from build123d import *

# Parameters (mm, degrees)
BOSS_EXTRUDE1_DEPTH = 31
SKETCH4_W           = 25
SKETCH4_H           = 15
CUT_EXTRUDE2_DEPTH  = 25
CUT_EXTRUDE4_DEPTH  = 11.5
SKETCH7_W           = 31
SKETCH7_H           = 1.7
BOSS_EXTRUDE3_DEPTH = 7
BOSS_EXTRUDE4_DEPTH = 7
LPATTERN1_COUNT     = 8
LPATTERN1_PITCH     = 3.6
SKETCH11_W          = 12
SKETCH11_H          = 4.5
BOSS_EXTRUDE5_DEPTH = 3.5
FILLET5_R           = 3
SKETCH12_W          = 12
SKETCH12_H          = 4.5
BOSS_EXTRUDE6_DEPTH = 4.5
CUT_EXTRUDE5_DEPTH  = 12


with BuildPart() as part:
    # Sketch1 → Boss-Extrude1 (new body)
    with BuildSketch(Plane.XY):
        Polygon((0, 0), (0, -30), (12, -30), (12, -20), (5, 0), align=None)
    extrude(amount=-BOSS_EXTRUDE1_DEPTH)

    # Sketch4 → Cut-Extrude2 (cut)
    with BuildSketch(Plane.ZY):
        with Locations((-15, -24.143402944)):
            Rectangle(SKETCH4_W, SKETCH4_H)
    extrude(amount=-CUT_EXTRUDE2_DEPTH, mode=Mode.SUBTRACT)

    # Sketch6 → Cut-Extrude4 (cut, symmetric)
    with BuildSketch(Plane.XY.offset(-15.25)):
        Polygon((5, 0), (5, -14), (9.9, -14), align=None)
    extrude(amount=CUT_EXTRUDE4_DEPTH, both=True, mode=Mode.SUBTRACT)

    # Sketch7 → Boss-Extrude3 (add)
    with BuildSketch(Plane(origin=(0, -27, 0), x_dir=(1, 0, 0), z_dir=(0, 1, 0))):
        with Locations((-4.2231607, 26.8)):
            Rectangle(SKETCH7_W, SKETCH7_H)
    extrude(amount=BOSS_EXTRUDE3_DEPTH)

    # Sketch10 → Boss-Extrude4 (add)
    with BuildSketch(Plane(origin=(0, -27, 0), x_dir=(1, 0, 0), z_dir=(0, 1, 0))):
        with BuildLine():
            Line((10.226247744, 22.144145979), (9.378053282, 22.144145979))
            ThreePointArc((9.378053282, 22.144145979), (8.729742796, 23.468564149), (8.93378471, 24.928960283))
            ThreePointArc((8.93378471, 24.928960283), (8.707970922, 25.446557347), (8.452150513, 25.95))
            Line((8.452150513, 25.95), (11.152150513, 25.95))
            ThreePointArc((11.152150513, 25.95), (10.896330104, 25.446557347), (10.670516315, 24.928960283))
            ThreePointArc((10.670516315, 24.928960283), (10.874558229, 23.468564149), (10.226247744, 22.144145979))
        make_face()
    boss_extrude4 = extrude(amount=BOSS_EXTRUDE4_DEPTH)

    # LPattern1: Boss-Extrude4 ×8
    with Locations(*[(-i * LPATTERN1_PITCH, 0, 0) for i in range(1, LPATTERN1_COUNT)]):
        add(boss_extrude4)

    # Sketch11 → Boss-Extrude5 (add)
    with BuildSketch(Plane(origin=(0, 0, -31), x_dir=(-1, 0, 0), z_dir=(0, 0, -1))):
        with Locations((-6, -27.75)):
            Rectangle(SKETCH11_W, SKETCH11_H)
    extrude(amount=BOSS_EXTRUDE5_DEPTH)

    # Fillet5
    fillet5_edges = [part.edges().sort_by_distance(p)[0] for p in [
        (5.412595515, -16.643402944, -27.5),
        (5.412595515, -16.643402944, -2.5),
        (5, -14, -15.25),
    ]]
    fillet(fillet5_edges, radius=FILLET5_R)

    # Sketch12 → Boss-Extrude6 (add)
    with BuildSketch(Plane.XY):
        with Locations((6, -27.75)):
            Rectangle(SKETCH12_W, SKETCH12_H)
    extrude(amount=BOSS_EXTRUDE6_DEPTH)

    # Sketch13 → Cut-Extrude5 (cut)
    with BuildSketch(Plane.ZY):
        Polygon((-33.25, -27.047861031), (-26.75, -27.047861031), (-26.75, -32.047861031), (-31.25, -32.047861031), (-31.25, -28.847861031), (-33.25, -28.847861031), align=None)
        Polygon((1.676178687, -28.847861031), (3.676178687, -28.847861031), (3.676178687, -27.047861031), (-2.823821313, -27.047861031), (-2.823821313, -32.047861031), (1.676178687, -32.047861031), align=None)
    extrude(amount=-CUT_EXTRUDE5_DEPTH, mode=Mode.SUBTRACT)


solid = part.part
Source: CAD feature listing. Evaluate the final solid. Frame: model axes, mm. A direction names the side the tool comes from. Round coordinates to 2 decimals unless told otherwise and drop trailing zeros. Loops run counter-clockwise (first coordinate to the right, second up) from the corner with the lowest first, then second, coordinate; pieces in that order, holes last. Notation, with made-up numbers: (25, 85) - (78, 85) arc R20 ccw to (78, 92) - close; hole circle Ø5 at (21, 12.5). An arc over 180 degrees is marked (long way). Write item = value, one per line. Start each with the question number.
(1) Ray query, line 1 along Z through (x, y) = (1, -20.75); line 2 along Z through (x, y) = (8, -11.5); line 3 along Y through (x, z) = (2, -21). Return the intervals inside material, ascending. Write a range as from..to.
(2) Pin query (flat end, axial travel): pin 1 (0.9 mm diameter, centred on x = -5, y = -24, fed in from +Z); pin 2 (2 mm diameter, centred on x = -1.5, y = -16.5, fed in from -Z) (3 decimals); pin 3 (1.5 mm diameter, centred on x = 7.5, y = -6, fed in from +Z); pin 4 (12 mm diameter, centred on y = -22, z = -18, fed in from -X). Return the tip coordinate at first contact, or that it passes through.
(3) Section query B-B, the plane z = -17. Output: boundary loops of the cut face in (x, y).
(4) Section query A-A, the plane y = -28. Output: boundary loops of the cut face in (x, z), plus the area to 3 significant figures.
(5) Set-up query: faces 1 (the face through (5, -5, -15)), 2 (the face through (6, -27.048, 1)), 3 (the face through (-16.49, -23.55, -25.44)). Return all of +Z, -Z, +X, -X, +Y, -Y with unobstructed straight access to the full face (end or side cutting, diameter ignored); none if empty.
(6) Pull-direction query (Z, two-part tool) for faces 4 (the face through (-10.722, -23.549, -23.489)), 5 (the face through (-10, -24, -27.65)), 6 (the face through (-13.6, -23.5, -25.95)), 7 (the face through (0, -12, -15)); classes: +Z half, -Z half, draft (parallel to the pull), parting line (faces both ways), or undercut.
(7) Section query C-C, the plane y = -9.25. Output: boundary loops of the cut face in (x, z), plus the area to 3 significant figures.
(8) Section query D-D, the plane y = -18.5. Output: boundary loops of the cut face in (x, z) (3 decimals).
Conclusion:
q1.line_1 = -31..-25.95, -2.5..0
q1.line_2 = -31..-26.75, -3.75..0
q1.line_3 = -16.64..0
q2.pin_1 = -22.14
q2.pin_2 = through
q2.pin_3 = 0
q2.pin_4 = -16.5
q3.outline = (0, -16.64) - (10.83, -16.64) - (9.9, -14) - (8, -14) arc R3 cw to (5, -11) - (5, 0) - (0, 0) - close
q4.outline = (0, -34.5) - (12, -34.5) - (12, -33.25) - (0, -33.25) - close; (0, 3.68) - (12, 3.68) - (12, 4.5) - (0, 4.5) - close
q4.area = 24.9 mm2
q5.face_1 = +X, +Y
q5.face_2 = +X, -X
q5.face_3 = -X, +Y, -Y
q6.face_4 = undercut
q6.face_5 = -Z half
q6.face_6 = +Z half
q6.face_7 = draft
q7.outline = (0, -31) - (8.24, -31) - (8.24, -26.75) - (5, -26.75) - (5, -3.75) - (8.24, -3.75) - (8.24, 0) - (0, 0) - close
q7.area = 181 mm2
q8.outline = (0, -31) - (11.475, -31) - (11.475, -27.274) - (0, -27.274) - close; (0, -2.726) - (11.475, -2.726) - (11.475, 0) - (0, 0) - close
